Drawing for the job (mm, zero at the part's lowest x, y, z). Coordinates: 2 decimals unless noted, no trailing zeros. Write each loop counter-clockwise with the first axis right and the second up, starting at its lowest first coordinate (ties: lowest second). Pieces come first, ordered by that corner, then holes. Notation, with made-up numbers: (1, -25.5) -> (51, -25.5) arc R16 ccw to (51, -16.5) -> close; hole circle Ø4 at (3.25, -0.5). An arc over 180 degrees is marked (long way). Answer as CSV lines item,"result".
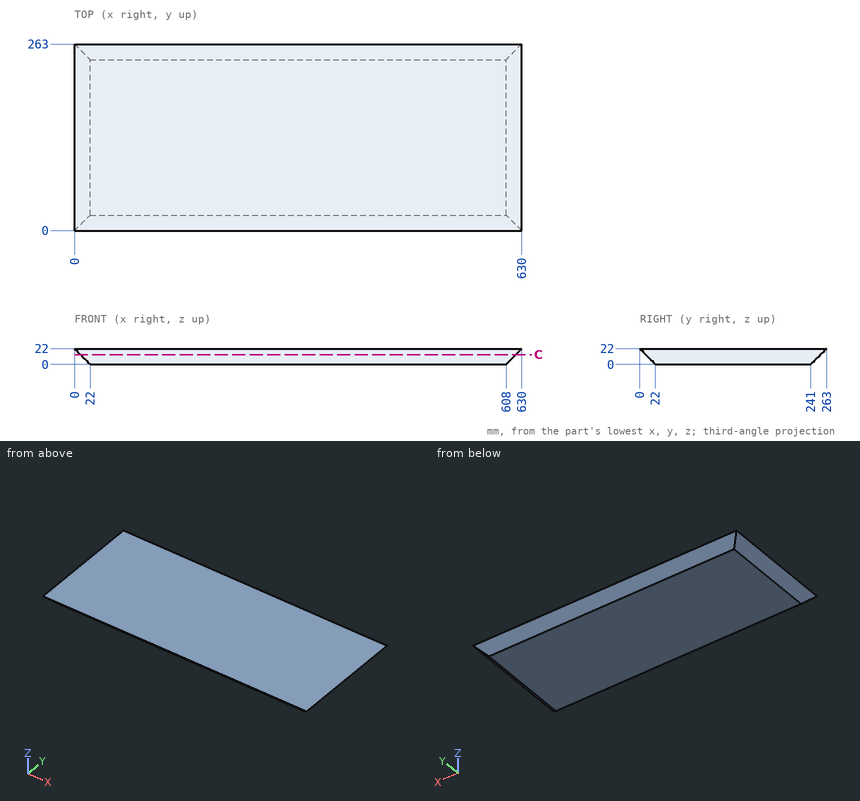
Item 1: Wall check: line 1 (Y direction, x = 405, z = 8); line 2 (Y direction, x = 369, z = 17.5); line 3 (Z direction, x = 389, y = 11.5). Give the ranges that are in metal, low to high. Write a range as from..to.
Answer below:
line 1,"y = 14..249"
line 2,"y = 4.5..258.5"
line 3,"z = 10.5..22"
Item 2: Saw through at C-C on z = 13.75. Give the cut face in (x, y), and give its area (3 significant figures).
Answer below:
outline,"(8.25, 8.25) -> (621.75, 8.25) -> (621.75, 254.75) -> (8.25, 254.75) -> close"
area,"151,000 mm2"
Item 3: Flat gauge pins, fed straight in: pin 1 (5 mm diameter, centred on x = 226, z = 10.5, fed in from -Y); pin 2 (6 mm diameter, centred on y = 108, z = 5, fed in from +X); pin 3 (10 mm diameter, centred on x = 567, z = 6.5, fed in from +Y). Where does each tip first touch, or does it go through?
Answer below:
pin 1,"stops at y = 9"
pin 2,"stops at x = 616"
pin 3,"stops at y = 252.5"
